Autodesk Fusion 360 part; units mm, degrees
sketch "Sketch1" plane through (0, 0, 0) normal (0, 1, 0) x (1, 0, 0)
  line L0 (0, 0) -> (-15, 0)
  spline S0 degree 5 poles (-15, 0) (-15, -2.4594) (-14.7958, -6.5576) (-13.8775, -10.2456) (-11.6701, -11.3146) (-8.3299, -11.1548) (-6.1225, -14.3711) (-5.2042, -21.1026) (-5, -27.9377) (-5, -31.9428) knots 0 0 0 0 0 0 0.2 0.4 0.6 0.8 1 1 1 1 1 1
  line L1 (-15, 5) -> (-15, -5)
  line L2 (0, 0) -> (0, -50)
  line L3 (-5, -23.8005) -> (-5, -40.085)
  line L4 (-5, -31.9428) -> (-6.6248, -31.4797)
  line L5 (-6.9086, -30.7495) -> (-5.0265, -28.8674)
  arc A0 (0, -30.5583) -> (0, -50) centre (0, -40.2791) ccw
  line L6 (-6.6248, -31.4797) -> (-6.9086, -30.7495)
  line L7 (-5.25, 0) -> (-5.25, -2.5)
  line L8 (-5.25, -2.5) -> (0, -2.5)
  dimension "d2" = 15
  dimension "d4" = 50
  dimension "d5" = 45
  dimension "d10" = 5
  dimension "d11" = 2.5
  dimension "d12" = 5.25
revolve "Revolve1" add sketch "Sketch1" angle 360 about axis through (0, 0, 0) along (0, 0, 1) contours L0 S0 L2 A0 L7 L8 | L2 A0 | S0 L4 L5 L6
equation "d2 = 1 / 2 * 3 cm"
Geometry check sheet. Reference: the model listing, model coordinates, mm. Coordinates: 2 decimals unless noted, no trailing zeros. Loops run counter-clockwise (first coordinate to the right, second up) from the corner with the lowest first, then second, coordinate; pieces in that order, holes last.
Item 1: Thickness scan on line 1 (Y direction, x = 0, z = 1); line 2 (X direction, y = 0, z = 1.45); line 3 (Z direction, x = -10.5, y = 4). Record the ranges inside material, lowest first.
Item 2: Go/stop test with flat-tipped pins: pin 1 Ø11.5 at (x, y) = (-0.5, -0.5) entering from -Z; pin 2 Ø8 at (y, z) = (-1.5, 34) entering from -X; pin 3 Ø6 at (x, y) = (-9.5, 6.5) entering from +Z; pin 4 Ø5 at (y, z) = (-1.5, 9) entering from +X. Record where each tip stops, or that it passes through.
Item 3: Release check for a two-part mould opening along Z. For faces 1 (the face through (0, 6, 0)), 2 (the face through (-4.91, -1.55, 28.99)), 3 (the face through (-5, -1.6, 1.3)) record: released by +Z, released by -Z, zero draft, split by the parting line, or undercut.
Item 4: Sectioned sample at A-A, the plane z = 37. Record the boundary of the cut face in (x, y), then the cut area to 3 significant figures.
Check result:
1. line 1: y = -14.99 to -5.25, 5.25 to 14.99
1. line 2: x = -14.98 to -5.25, 5.25 to 14.98
1. line 3: z = 0 to 11.04
2. pin 1: stops at z = 0
2. pin 2: stops at x = -9.41
2. pin 3: stops at z = 44.98
2. pin 4: stops at x = 14.5
3. face 1: released by -Z
3. face 2: undercut
3. face 3: zero draft
4. outline: circle Ø18.3 at (0, 0)
4. area: 263 mm2
